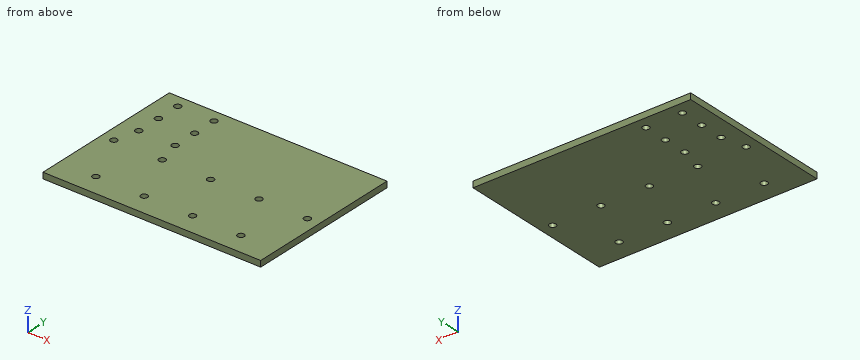
Autodesk Inventor part; units mm, degrees
ref_plane "YZ Plane" through (0, 0, 0) normal (1, 0, 0) x (0, 1, 0)
ref_plane "XZ Plane" through (0, 0, 0) normal (0, 1, 0) x (-1, 0, 0)
ref_plane "XY Plane" through (0, 0, 0) normal (0, 0, 1) x (1, 0, 0)
sketch "Sketch1" plane through (0, 0, 0) normal (0, 0, 1) x (1, 0, 0)
  line L0 (0, 0) -> (180, 0)
  line L1 (180, 0) -> (180, -130)
  line L2 (180, -130) -> (0, -130)
  line L3 (0, -130) -> (0, 0)
  dimension "d0" = 180
  dimension "d1" = 130
extrude "Extrusion1" add sketch "Sketch1" along normal blind 5
sketch "Sketch2" plane through (0, 0, 5) normal (0, 0, 1) x (1, 0, 0)
  line L0 (0, -130) -> (180, -130)
  line L1 (180, -130) -> (150, -130)
  line L2 (150, -130) -> (150, -113)
  circle A0 centre (150, -113) radius 2.75
  line L3 (180, -130) -> (180, 0)
  line L4 (180, -69.5) -> (170, -69.5)
  line L5 (180, -69.5) -> (190, -69.5) construction
  circle A1 centre (170, -69.5) radius 2.75
  circle A2 centre (130, -69.5) radius 2.75
  circle A3 centre (90, -69.5) radius 2.75
  circle A4 centre (50, -69.5) radius 2.75
  circle A5 centre (10, -69.5) radius 2.75
  circle A6 centre (110, -113) radius 2.75
  circle A7 centre (70, -113) radius 2.75
  circle A8 centre (30, -113) radius 2.75
  point P0 (0, 0)
  dimension "d4" = 30
  dimension "d6" = 5.5
  dimension "d25" = 10
  dimension "d26" = 180
  dimension "d33" = 5.5
  dimension "d34" = 5.5
  dimension "d35" = 5.5
  dimension "d37" = 5.5
  dimension "d53" = 43.5
  dimension "d56" = 40
extrude "Extrusion2" cut sketch "Sketch2" against normal blind 5
sketch "Sketch3" plane through (0, 0, 5) normal (0, 0, 1) x (1, 0, 0)
  line L0 (0, 0) -> (180, 0)
  line L1 (0, 0) -> (15, 0)
  line L2 (15, 0) -> (15, -10)
  circle A0 centre (15, -10) radius 2.75
  line L3 (15, -10) -> (15, -30)
  line L4 (15, -30) -> (15, -50)
  circle A1 centre (15, -30) radius 2.75
  circle A2 centre (15, -50) radius 2.75
  line L5 (15, -10) -> (45, -10)
  line L6 (45, -10) -> (45, -30)
  line L7 (45, -30) -> (45, -50)
  circle A3 centre (45, -10) radius 2.75
  circle A4 centre (45, -30) radius 2.75
  circle A5 centre (45, -50) radius 2.75
  dimension "d40" = 15
  dimension "d41" = 10
  dimension "d42" = 5.5
  dimension "d43" = 20
  dimension "d44" = 20
  dimension "d45" = 5.5
  dimension "d46" = 5.5
  dimension "d47" = 30
  dimension "d48" = 5.5
  dimension "d49" = 5.5
  dimension "d50" = 5.5
extrude "Extrusion3" cut sketch "Sketch3" against normal blind 5
properties part number "GantryPlate_v3"
For this review, take the finished solid that the model builds, in its own axes (mm). Give positions to 0.01 mm unless a question says otherwise; leave off trailing zeros. Order: outer loops, then holes, each group sorted by start corner. A loop starts at its lowest first (then second) coordinate and runs counter-clockwise, first axis right, second up.
1) Insertion check: pin 1 (6.5 mm diameter, centred on x = 170, y = -69.5, fed in from +Z). The pin has a flat end and moves straight along its axis. Give the tip position at first contact, or say it passes through.
2) Wall thickness on line 1 (X direction, y = -10, z = 1.1); line 2 (Y direction, x = 45, z = 3); line 3 (Y direction, x = 70, z = 3.8): over which ranges is each line inside the solid? List them lowest first.
3) Take a section at B-B (z = 2.05). State how many separate pieces and enclosed holes the cut face has, then the cut area to 3 significant figures.
4) Take a section at C-C (x = 170). Give the boundary of the cut face in (y, z).
5) Take a section at D-D (y = -50). Give the boundary of the cut face in (x, z), then the cut area to 3 significant figures.
6) Take a section at A-A (y = -69.5). Give the boundary of the cut face in (x, z), then the cut area to 4 significant figures.
Derived:
1. pin 1: stops at z = 5
2. line 1: x = 0 to 12.25, 17.75 to 42.25, 47.75 to 180
2. line 2: y = -130 to -52.75, -47.25 to -32.75, -27.25 to -12.75, -7.25 to 0
2. line 3: y = -130 to -115.75, -110.25 to 0
3. separate pieces: 1
3. enclosed holes: 15
3. area: 23,000 mm2
4. outline: (-130, 0) - (-72.25, 0) - (-72.25, 5) - (-130, 5) - close; (-66.75, 0) - (0, 0) - (0, 5) - (-66.75, 5) - close
5. outline: (0, 0) - (12.25, 0) - (12.25, 5) - (0, 5) - close; (17.75, 0) - (42.25, 0) - (42.25, 5) - (17.75, 5) - close; (47.75, 0) - (180, 0) - (180, 5) - (47.75, 5) - close
5. area: 845 mm2
6. outline: (0, 0) - (7.25, 0) - (7.25, 5) - (0, 5) - close; (12.75, 0) - (47.25, 0) - (47.25, 5) - (12.75, 5) - close; (52.75, 0) - (87.25, 0) - (87.25, 5) - (52.75, 5) - close; (92.75, 0) - (127.25, 0) - (127.25, 5) - (92.75, 5) - close; (132.75, 0) - (167.25, 0) - (167.25, 5) - (132.75, 5) - close; (172.75, 0) - (180, 0) - (180, 5) - (172.75, 5) - close
6. area: 762.5 mm2
